```python
from build123d import *

# Parameters (mm, degrees)
F1_DEPTH = 50
F3_DEPTH = 100
F4_R     = 2.5
F5_DEPTH = 5


with BuildPart() as f1:
    # F0 (on Right) → F1 (new body, symmetric)
    with BuildSketch(Plane.YZ):
        Polygon((-64.5, 0), (0, 0), (0, 12), (-4.5, 12), (-4.5, 5), (-64.5, 5), align=None)
    extrude(amount=F1_DEPTH, both=True)

    # F2 (on face) → F3 (cut, through all)
    with BuildSketch(Plane.YZ.offset(50)):
        Polygon((0, 12), (-2.25, 12), (0, 4.411913), align=None)
    extrude(amount=-F3_DEPTH, mode=Mode.SUBTRACT)

    # F4 (on face) → F5 (cut, through all)
    with BuildSketch(Plane.XY.offset(5)):
        with Locations((-30, -39.5)):
            Circle(F4_R)
        with Locations((30, -39.5)):
            Circle(F4_R)
    extrude(amount=-F5_DEPTH, mode=Mode.SUBTRACT)


solid = f1.part
```
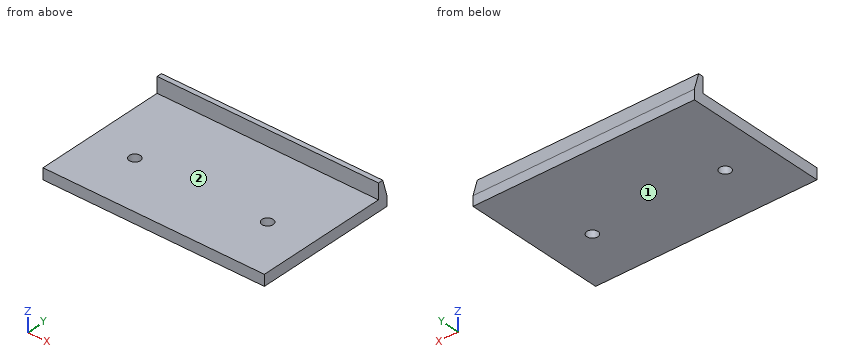
Verification items for the finished model (mm, model axes). Face numbers are marked on the shaded views. A direction names the side the tool comes from. Give positions to 0.01 mm unless a question says otherwise; leave off trailing zeros. Loops run counter-clockwise (first coordinate to the right, second up) from the corner with the lowest first, then second, coordinate; pieces in that order, holes last. Notation, with made-up numbers: M 21,72 L 34,72 A11 ccw 34,80 Z; hole C 3,-34.5 d3. An arc over 180 degrees is marked long. Return JSON: item names as keys, results as strings.
1) Gauge pin test, flat ends, axial feed: P1, Ø1.5, axis at x = -0.5, z = 6, coming from the +Y side; P2, Ø5, axis at x = -39, z = 2, coming from the +Y side; P3, Ø6, axis at x = 37, y = -26, coming from the +Z side; P4, Ø3.5, axis at x = 0.5, z = 8, coming from the -Y side. Record the tip position at first contact, or that the pin passes through.
Findings:
{"P1": "stops at y = -0.25", "P2": "stops at y = 0", "P3": "stops at z = 5", "P4": "stops at y = -4.5"}
2) Section check D-D, the plane y = -18. Enter the section's corners in (x, z).
Findings:
{"outline": "M -50,0 L 50,0 L 50,5 L -50,5 Z"}
3) Material ranges on L1, parallel to Y at x = 30, z = 1.9; L2, parallel to Z at x = -23, y = -21.5; L3, parallel to X at y = -38, z = 4.75, recorded low to high. Write a range as [from, to].
Findings:
{"L1": "y = [-64.5, -42], [-37, 0]", "L2": "z = [0, 5]", "L3": "x = [-50, -32], [-28, 28], [32, 50]"}
4) Section check B-B, the plane y = -39.5. Enter the section's corners in (x, z), and give its area (3 significant figures).
Findings:
{"outline": "M -50,0 L -32.5,0 L -32.5,5 L -50,5 Z; M -27.5,0 L 27.5,0 L 27.5,5 L -27.5,5 Z; M 32.5,0 L 50,0 L 50,5 L 32.5,5 Z", "area": "450 mm2"}
5) Tool access check on the marked faces 1 and 2. Record the directions out of +Z, -Z, +X, -X, +Y, -Y that give a thin tool (end or side, any length) a straight path to the whole face; none if there is none.
Findings:
{"face 1": "-Z, +X, -X, +Y, -Y", "face 2": "+Z, +X, -X, -Y"}
6) Section check C-C, the plane x = -34. Enter the section's corners in (y, z), and give its area (3 significant figures).
Findings:
{"outline": "M -64.5,0 L 0,0 L 0,4.41 L -2.25,12 L -4.5,12 L -4.5,5 L -64.5,5 Z", "area": "345 mm2"}
7) Section check A-A, the plane x = 30. Enter the section's corners in (y, z).
Findings:
{"outline": "M -64.5,0 L -42,0 L -42,5 L -64.5,5 Z; M -37,0 L 0,0 L 0,4.41 L -2.25,12 L -4.5,12 L -4.5,5 L -37,5 Z"}
